For this review, take the finished solid that the model builds, in its own axes (mm). Face numbers are marked on the shaded views. A direction names the side the tool comes from. Give positions to 0.01 mm unless a question says otherwise; leave off trailing zeros. Order: outer loops, then holes, each group sorted by start corner. A loop starts at its lowest first (then second) coordinate and runs counter-clockwise, first axis right, second up. Notation, with made-up numbers: (10.25, -25) - (26.25, -25) arc R20 ccw to (26.25, 11) - close; hole circle Ø8 at (-32, 25.5). An arc over 180 degrees is marked (long way). Use a Markdown table: item, result. Add a question column.
1) We need section B-B on x = -3.5. Write out the cut boundary in (y, z).
2) Clearance check with flat-ended pins moving along their axes: P1, Ø8, axis at y = -3, z = -14.5, coming from the -X side; P2, Ø1, axis at x = -6.5, z = 16.5, coming from the +Y side; P3, Ø1.7, axis at x = 6.5, y = 8.5, coming from the +Z side. State where each tip first meets the part, or that it passes through.
3) We need section A-A on y = 0. Write out the cut boundary in (x, z).
4) We need section C-C on z = -7.5. Write out the cut boundary in (x, y), then the cut area to 3 significant figures.
5) Machinability: for the marked faces 1, 2, 3, 4 and 5, which of the approach directions +Z, -Z, +X, -X, +Y, -Y give a long, thin tool a straight path to every point of the face, cutting with its end or side? Answer none if there is none.
6) We need section D-D on y = -7.75. Write out the cut boundary in (x, z).
7) Wall thickness on L1, parallel to X at y = -0.25, z = 15; L2, parallel to Y at x = 0, z = -2; L3, parallel to X at y = -2.25, z = -17.5: over which ranges is each line inside the solid? List them lowest first.
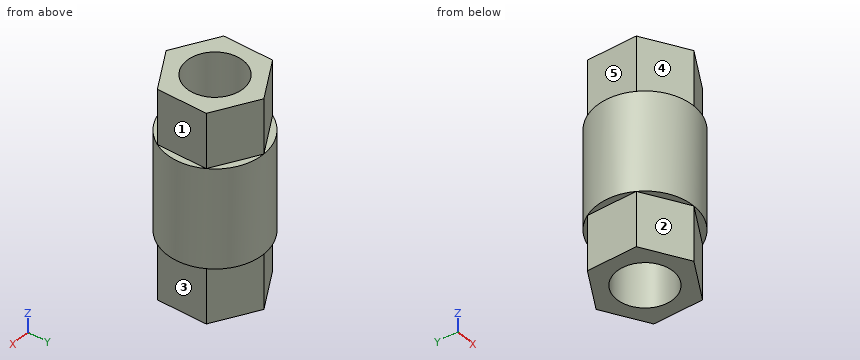
```python
from build123d import *

# Parameters (mm, degrees)
SKETCH1_R           = 11
SKETCH1_R_2         = 6.4
BOSS_EXTRUDE1_DEPTH = 11.4
SKETCH1_3_R         = 6.4
BOSS_EXTRUDE2_DEPTH = 24


with BuildPart() as part:
    # Sketch1 → Boss-Extrude1 (new body, symmetric)
    with BuildSketch(Plane.XY):
        Circle(SKETCH1_R)
        Circle(SKETCH1_R_2, mode=Mode.SUBTRACT)
    extrude(amount=BOSS_EXTRUDE1_DEPTH, both=True)

    # Sketch1_3 → Boss-Extrude2 (add, symmetric)
    with BuildSketch(Plane.XY):
        Polygon((-9.526279442, 5.5), (-9.526279442, -5.5), (0, -11), (9.526279442, -5.5), (9.526279442, 5.5), (0, 11), align=None)
        Circle(SKETCH1_3_R, mode=Mode.SUBTRACT)
    extrude(amount=BOSS_EXTRUDE2_DEPTH, both=True)


solid = part.part
```
Checked values:
| question | item | result |
|---|---|---|
| 1 | outline | (-10.43, -11.4) - (-8.98, -11.4) - (-8.98, -24) - (-5.36, -24) - (-5.36, 24) - (-8.98, 24) - (-8.98, 11.4) - (-10.43, 11.4) - close; (5.36, -24) - (8.98, -24) - (8.98, -11.4) - (10.43, -11.4) - (10.43, 11.4) - (8.98, 11.4) - (8.98, 24) - (5.36, 24) - close |
| 2 | P1 | x = -10.99 |
| 2 | P2 | y = 7.54 |
| 2 | P3 | z = 11.4 |
| 3 | outline | (-11, -11.4) - (-9.53, -11.4) - (-9.53, -24) - (-6.4, -24) - (-6.4, 24) - (-9.53, 24) - (-9.53, 11.4) - (-11, 11.4) - close; (6.4, -24) - (9.53, -24) - (9.53, -11.4) - (11, -11.4) - (11, 11.4) - (9.53, 11.4) - (9.53, 24) - (6.4, 24) - close |
| 4 | outline | circle Ø22 at (0, 0); hole circle Ø12.8 at (0, 0) |
| 4 | area | 251 mm² |
| 5 | face 1 | +Z, +X, +Y, -Y |
| 5 | face 2 | -Z, -X, -Y |
| 5 | face 3 | -Z, +X, +Y, -Y |
| 5 | face 4 | +Z, -X, -Y |
| 5 | face 5 | +Z, -X, +Y, -Y |
| 6 | outline | (-7.81, -11.4) - (-5.63, -11.4) - (-5.63, -24) - (5.63, -24) - (5.63, -11.4) - (7.81, -11.4) - (7.81, 11.4) - (5.63, 11.4) - (5.63, 24) - (-5.63, 24) - (-5.63, 11.4) - (-7.81, 11.4) - close |
| 7 | L1 | -9.53 to -6.4, 6.4 to 9.53 |
| 7 | L2 | -11 to -6.4, 6.4 to 11 |
| 7 | L3 | -9.53 to -5.99, 5.99 to 9.53 |
